Check sheet for the modelled part. Datum: model origin and axes. Units: mm. A direction names the side the tool comes from. Round coordinates to 2 decimals unless told otherwise and drop trailing zeros. Order: outer loops, then holes, each group sorted by start corner. A loop starts at its lowest first (then second) coordinate and runs counter-clockwise, first axis right, second up. Notation, with made-up numbers: (35.25, 77.25) -> (75.25, 77.25) arc R33 ccw to (75.25, 115.25) -> close; hole circle Ø4 at (-18.5, 49.5). An arc over 180 degrees is marked (long way). Answer in a Markdown table with one row per item.
from build123d import *

# Parameters (mm, degrees)
CYLINDER_R      = 20
CYLINDER_DEPTH  = 3.3
SKETCH_R        = 1.5
POCKET_DEPTH    = 3.301
POCKET001_DEPTH = 3.301


with BuildPart() as part:
    # Cylinder → Cylinder (new body)
    with BuildSketch(Plane.XY):
        Circle(CYLINDER_R)
    extrude(amount=CYLINDER_DEPTH)

    # Sketch → Pocket (cut, through all)
    with BuildSketch(Plane.XY.offset(3.3)):
        with Locations((0, 15.1)):
            Circle(SKETCH_R)
    extrude(amount=-POCKET_DEPTH, mode=Mode.SUBTRACT)

    # Sketch001 → Pocket001 (cut, through all)
    with BuildSketch(Plane(origin=(0, 0, 0), x_dir=(1, 0, 0), z_dir=(0, 0, -1))):
        Polygon((12.641277, -8.466407), (-12.641277, -8.466407), (0.000337, 15.21453), align=None)
    extrude(amount=-POCKET001_DEPTH, mode=Mode.SUBTRACT)


solid = part.part
Item 1: Cross-section at B-B (x = -6). Record the boundary of the cut face in (y, z), and give its area (3 significant figures).
Result sheet:
| item | result |
|---|---|
| outline | (-19.08, 0) -> (-3.97, 0) -> (-3.97, 3.3) -> (-19.08, 3.3) -> close; (8.47, 0) -> (19.08, 0) -> (19.08, 3.3) -> (8.47, 3.3) -> close |
| area | 84.9 mm^2 |
Item 2: Set-up check for faces 4 (the flat face through (9, 0, 0)), 5 (the flat face through (0, 8.466, 2)): record each of +Z, -Z, +X, -X, +Y, -Y from which the full face is reachable in a straight line by a thin tool's end or side.
Result sheet:
| item | result |
|---|---|
| face 4 | -Z, +X, -X, +Y, -Y |
| face 5 | +Z, -Z |
Item 3: Mould release check, pull along X, two halves, no side actions. Record for faces 1 (the flat face through (9, 0, 3.3)), 2 (the flat face through (6.23, -3.54, 1.63)), 3 (the cylindrical face through (-4.336, -19.524, 1.627)): pulls with the +X half, pulls with the -X half, needs draft (parallel to the pull), parting line crosses it, or undercut.
Result sheet:
| item | result |
|---|---|
| face 1 | needs draft |
| face 2 | undercut |
| face 3 | parting line crosses it |
Item 4: Cross-section at C-C (z = 2.6). Record the boundary of the cut face in (x, y).
Result sheet:
| item | result |
|---|---|
| outline | circle Ø40 at (0, 0); hole (-12.64, 8.47) -> (0, -15.21) -> (12.64, 8.47) -> close; hole circle Ø3 at (0, 15.1) |
Item 5: Cross-section at D-D (x = 15). Record the boundary of the cut face in (y, z).
Result sheet:
| item | result |
|---|---|
| outline | (-13.23, 0) -> (13.23, 0) -> (13.23, 3.3) -> (-13.23, 3.3) -> close |
Item 6: Cross-section at A-A (y = -2.5). Record the boundary of the cut face in (x, z).
Result sheet:
| item | result |
|---|---|
| outline | (-19.84, 0) -> (-6.79, 0) -> (-6.79, 3.3) -> (-19.84, 3.3) -> close; (6.79, 0) -> (19.84, 0) -> (19.84, 3.3) -> (6.79, 3.3) -> close |
Item 7: Scan lines: line 1 (X direction, y = -4, z = 2.75); line 2 (X direction, y = 2, z = 2.9); line 3 (Y direction, x = -1, z = 3.15). Record each from-to range of solid material in increasing order. Write a range as [from, to].
Result sheet:
| item | result |
|---|---|
| line 1 | x = [-19.6, -5.99], [5.99, 19.6] |
| line 2 | x = [-19.9, -9.19], [9.19, 19.9] |
| line 3 | y = [-19.97, -13.34], [8.47, 13.98], [16.22, 19.97] |
Item 8: Depth check by flat-ended pin: P1, Ø1, axis at x = 3, z = 2, coming from the -Y side; P2, Ø2.5, axis at x = 0, y = 15.1, coming from the -Z side; P3, Ø1.5, axis at y = 14.5, z = 3, coming from the -X side; P4, Ø1, axis at x = 2, z = 0.5, coming from the +Y side. Enter the tip coordinate at first touch or a pass-through.
Result sheet:
| item | result |
|---|---|
| P1 | stops at y = -19.84 |
| P2 | passes through |
| P3 | stops at x = -14.52 |
| P4 | stops at y = 19.94 |
